Geometry check sheet. Reference: drawing and pictorial views, mm from the part's lowest x, y, z. A direction names the side the tool comes from. Round coordinates to 2 decimals unless told otherwise and drop trailing zeros. Write each loop counter-clockwise with the first axis right and the second up, starting at its lowest first coordinate (ties: lowest second). Pieces come first, ordered by that corner, then holes.
Item 1: Depth check by flat-ended pin: pin 1 (2 mm diameter, centred on x = 6, z = 9.5, fed in from -Y); pin 2 (2 mm diameter, centred on x = 6, z = 9.5, fed in from +Y); pin 3 (1.5 mm diameter, centred on x = 2.5, z = 14, fed in from +Y). Enter the tip coordinate at first touch or a pass-through.
Item 2: Section check D-D, the plane z = 2.25. Record the cut outline in (x, y), plus the area to 3 significant figures.
Item 3: Section check C-C, the plane z = 15. Record the cut outline in (x, y).
Item 4: Section check A-A, the plane x = 4. Record the cut outline in (y, z), plus the area to 3 significant figures.
Item 5: Set-up check for the marked faces 1, 2 and 3: record each of +Z, -Z, +X, -X, +Y, -Y from which the full face is reachable in a straight line by a thin tool's end or side.
Item 6: Material ranges on line 1 along Z through (x, y) = (3.25, 2); line 2 along Z through (x, y) = (5.75, 1); line 3 along Y through (x, z) = (2.25, 11), recorded low to high.
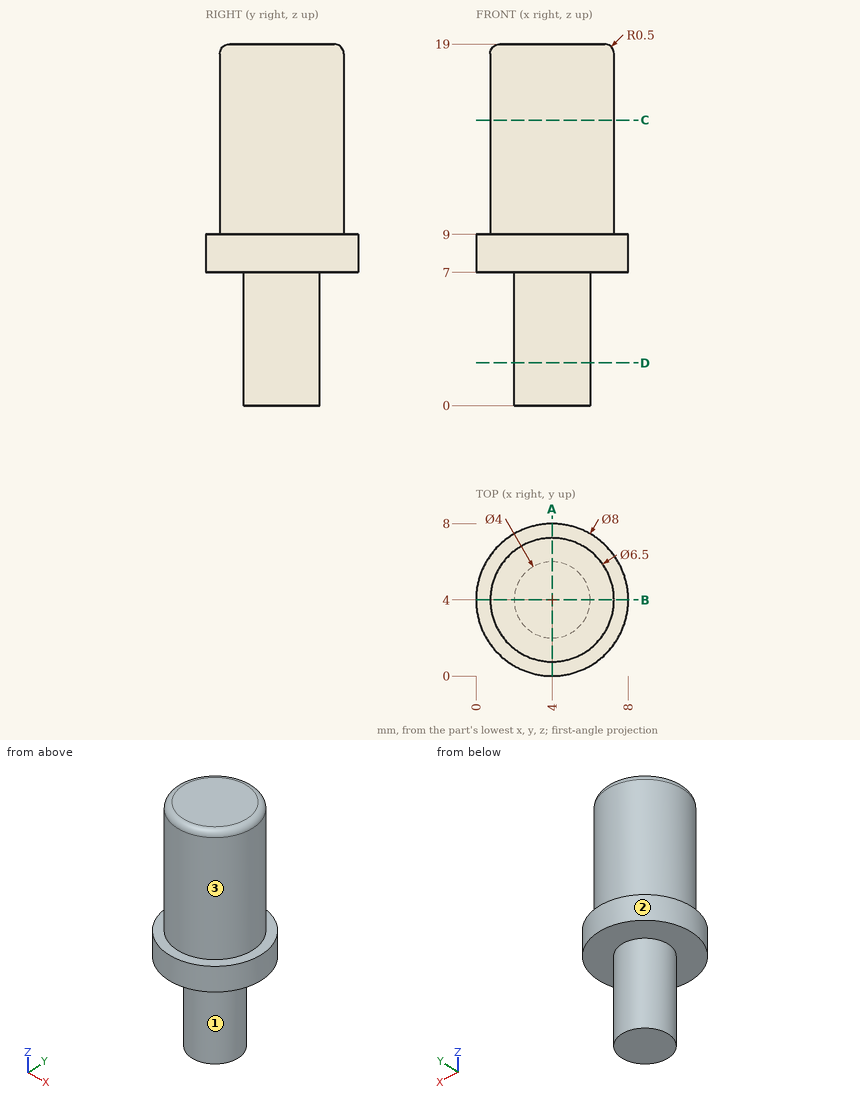
Values found:
1. pin 1: stops at y = 0.16
1. pin 2: stops at y = 7.84
1. pin 3: stops at y = 7.16
2. outline: circle Ø4 at (4, 4)
2. area: 12.6 mm2
3. outline: circle Ø6.5 at (4, 4)
4. outline: (0, 7) - (2, 7) - (2, 0) - (6, 0) - (6, 7) - (8, 7) - (8, 9) - (7.25, 9) - (7.25, 18.5) arc R0.5 ccw to (6.75, 19) - (1.25, 19) arc R0.5 ccw to (0.75, 18.5) - (0.75, 9) - (0, 9) - close
4. area: 109 mm2
5. face 1: -Z
5. face 2: +Z, -Z
5. face 3: +Z
6. line 1: z = 7 to 19
6. line 2: z = 7 to 9
6. line 3: y = 1.26 to 6.74
